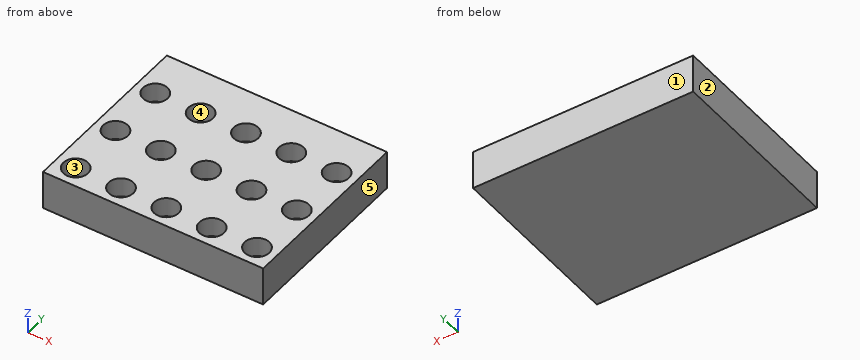
Solid Edge part; units mm, degrees
sketch "Sketch1" plane through (0, 0, 0) normal (0, 0, 1) x (1, 0, 0)
  line L0 (-85, -70) -> (85, -70)
  line L1 (85, -70) -> (85, 70)
  line L2 (85, 70) -> (-85, 70)
  line L3 (-85, 70) -> (-85, -70)
extrude "Protrusion1" add sketch "Sketch1" against normal blind 30
sketch "Sketch2" plane through (0, 0, 0) normal (0, 0, 1) x (1, 0, 0)
  circle A0 centre (-70, -55) radius 9.5
  circle A1 centre (-35, -55) radius 9.5
  circle A2 centre (0, -55) radius 9.5
  circle A3 centre (35, -55) radius 9.5
  circle A4 centre (70, -55) radius 9.5
  circle A5 centre (70, -10) radius 9.5
  circle A6 centre (70, 35) radius 9.5
  circle A7 centre (35, -10) radius 9.5
  circle A8 centre (0, -10) radius 9.5
  circle A9 centre (-35, -10) radius 9.5
  circle A10 centre (-70, -10) radius 9.5
  circle A11 centre (35, 35) radius 9.5
  circle A12 centre (0, 35) radius 9.5
  circle A13 centre (-35, 35) radius 9.5
  circle A14 centre (-70, 35) radius 9.5
extrude "Recorte_Extrudado_1" cut sketch "Sketch2" against normal blind 15
Can you work these out from the model? Positions are in its coordinate system, mm. Face numbers are marked on the shaded views. A direction names the side the tool comes from. Coordinates: 2 decimals unless noted, no trailing zeros. Write each loop counter-clockwise with the first axis right and the second up, starting at its lowest first coordinate (ties: lowest second). Pieces come first, ordered by that corner, then holes. Notation, with made-up numbers: (76.25, 11.5) -> (81.25, 11.5) arc R14 cw to (81.25, 15.5) -> close; hole circle Ø6 at (-8, -30.5). An arc over 180 degrees is marked (long way). Write each question's results on one line, items separated by ' | '. Start each with the question number.
Item 1: I'm going to push a flat-ended pin straight in: P1, Ø5.5, axis at x = 67, y = -13.5, coming from the +Z side. Where does the tip first touch, or does it pass through?
Item 2: On a 3-axis mill with a long thin cutter (end or side, diameter ignored), from which of +Z, -Z, +X, -X, +Y, -Y can I reach the whole of each face in a straight line? I mean the marked faces 4 and 5. Say none if no direction works.
Item 3: If we section it at A-A, the plane y = 35: Write out the boundary of the cut face in (x, z), and give its area (4 significant figures).
Item 4: Thinking about a two-plate mould opening in X: for the marked faces 1, 2 and 3, which applies, released by +X, released by -X, zero draft, split by the parting line, or undercut?
Item 5: If we section it at C-C, the plane x = 0: Write out the boundary of the cut face in (y, z).
Item 6: Please list where these lines run through material, in increasing order: probe 1 along Y at (x, z) = (70, -6.5); probe 2 along X at (y, z) = (-13, -12.5); probe 3 along Y at (x, z) = (-63, -12.75).
Item 7: If we section it at D-D, the plane x = -66.5: Write out the boundary of the cut face in (y, z), and give its area (3 significant figures).
Item 8: If we section it at B-B, the plane z = -6.75: Count the separate pieces of the cut face and the enclosed holes in it, and give its area (3 significant figures).
Answer block:
1) P1: z = -15
2) face 4: +Z | face 5: +Z, -Z, +X, +Y, -Y
3) outline: (-85, -30) -> (85, -30) -> (85, 0) -> (79.5, 0) -> (79.5, -15) -> (60.5, -15) -> (60.5, 0) -> (44.5, 0) -> (44.5, -15) -> (25.5, -15) -> (25.5, 0) -> (9.5, 0) -> (9.5, -15) -> (-9.5, -15) -> (-9.5, 0) -> (-25.5, 0) -> (-25.5, -15) -> (-44.5, -15) -> (-44.5, 0) -> (-60.5, 0) -> (-60.5, -15) -> (-79.5, -15) -> (-79.5, 0) -> (-85, 0) -> close | area: 3,675 mm²
4) face 1: zero draft | face 2: released by -X | face 3: undercut
5) outline: (-70, -30) -> (70, -30) -> (70, 0) -> (44.5, 0) -> (44.5, -15) -> (25.5, -15) -> (25.5, 0) -> (-0.5, 0) -> (-0.5, -15) -> (-19.5, -15) -> (-19.5, 0) -> (-45.5, 0) -> (-45.5, -15) -> (-64.5, -15) -> (-64.5, 0) -> (-70, 0) -> close
6) probe 1: -70 to -64.5, -45.5 to -19.5, -0.5 to 25.5, 44.5 to 70 | probe 2: -85 to -79.01, -60.99 to -44.01, -25.99 to -9.01, 9.01 to 25.99, 44.01 to 60.99, 79.01 to 85 | probe 3: -70 to -61.42, -48.58 to -16.42, -3.58 to 28.58, 41.42 to 70
7) outline: (-70, -30) -> (70, -30) -> (70, 0) -> (43.83, 0) -> (43.83, -15) -> (26.17, -15) -> (26.17, 0) -> (-1.17, 0) -> (-1.17, -15) -> (-18.83, -15) -> (-18.83, 0) -> (-46.17, 0) -> (-46.17, -15) -> (-63.83, -15) -> (-63.83, 0) -> (-70, 0) -> close | area: 3,410 mm²
8) separate pieces: 1 | enclosed holes: 15 | area: 19,500 mm²
